Geometry check sheet. Reference: the model listing, model coordinates, mm. A direction names the side the tool comes from. Give positions to 0.01 mm unless a question says otherwise; leave off trailing zeros. Loops run counter-clockwise (first coordinate to the right, second up) from the corner with the lowest first, then second, coordinate; pieces in that order, holes last. Notation, with made-up numbers: (-4.5, -7) -> (34.5, -7) arc R23 ccw to (34.5, 20) -> close; hole circle Ø6 at (-21.75, 44.25). An arc over 180 degrees is marked (long way). One line per question, with ' | ' between items.
from build123d import *


with BuildPart() as part:
    # ｽｲｰﾌﾟ1: sweep along a path in ｽｹｯﾁ2
    with BuildLine(Plane.XY) as sweep_1_path:
        Line((0, -13.345), (-431, -13.345))
        ThreePointArc((-431, -13.345), (-444.345, 0), (-431, 13.345))
        Line((-431, 13.345), (0, 13.345))
        ThreePointArc((0, 13.345), (13.345, 0), (0, -13.345))
    # Sketch 3D_3 → ｽｲｰﾌﾟ1 (sweep)
    with BuildSketch(Plane(origin=(0, 13.345, 0), x_dir=(-1.3735006890805393e-13, 0.29124620867342393, -0.956648130679905), z_dir=(1, 0, 0))):
        Polygon((0, 0), (4.304916588, -1.310607939), (4.703923894, 0), (-3.905909282, 2.621215878), (-4.304916588, 1.310607939), align=None)
    sweep(path=sweep_1_path.line)


solid = part.part
Item 1: Sectioned sample at A-A (y = 0). Record the cut outline in (x, z) (3 decimals).
Result:
outline: (-445.715, -4.5) -> (-444.345, -4.5) -> (-444.345, 4.5) -> (-445.715, 4.5) -> close; (13.345, -4.5) -> (14.715, -4.5) -> (14.715, 4.5) -> (13.345, 4.5) -> close
Item 2: Sectioned sample at B-B (x = -126). Record the cut outline in (y, z) (3 decimals), plus the area to 3 significant figures.
Result:
outline: (-14.715, -4.5) -> (-13.345, -4.5) -> (-13.345, 4.5) -> (-14.715, 4.5) -> close; (13.345, -4.5) -> (14.715, -4.5) -> (14.715, 4.5) -> (13.345, 4.5) -> close | area: 24.7 mm2
Item 3: Sectioned sample at C-C (z = 1.5). Record the cut outline in (x, y) (3 decimals), plus the area to 3 significant figures.
Result:
outline: (-431, -14.715) -> (0, -14.715) arc R14.715 ccw to (0, 14.715) -> (-431, 14.715) arc R14.715 ccw to start; hole (-431, -13.345) -> (0, -13.345) arc R13.345 ccw to (0, 13.345) -> (-431, 13.345) arc R13.345 ccw to start | area: 1,300 mm2
Item 4: Release check for a two-part mould opening along Y. For faces 1 (the face through (-445.71, -0.32, 0.06)), 2 (the face through (-219, -14.715, 0)), 3 (the face through (-444.34, -0.29, -0.06)), 4 (the face through (-212, 14.715, 0)) record: pulls with the +Y half, pulls with the -Y half, needs draft (parallel to the pull), parting line crosses it, or undercut.
Result:
face 1: parting line crosses it | face 2: pulls with the -Y half | face 3: undercut | face 4: pulls with the +Y half
Item 5: Scan lines: probe 1 along Y at (x, z) = (-26.5, 1.5) (3 decimals); probe 2 along X at (y, z) = (1.5, 2.5); probe 3 along X at (y, z) = (-9.5, 0). Record each from-to range of solid material in increasing order.
Result:
probe 1: -14.715 to -13.345, 13.345 to 14.715 | probe 2: -445.64 to -444.26, 13.26 to 14.64 | probe 3: -442.24 to -440.37, 9.37 to 11.24
Item 6: Set-up check for faces 5 (the face through (13.34, 0.29, -0.06)), 6 (the face through (14.71, 0.32, 0.06)): record each of +Z, -Z, +X, -X, +Y, -Y from which the full face is reachable in a straight line by a thin tool's end or side.
Result:
face 5: +Z, -Z | face 6: +Z, -Z, +X
